```python
from build123d import *

# Parameters (mm, degrees)
F_3_0MM_DOWEL_HOLE1_D           = 3
F_3_0MM_DOWEL_HOLE1_ON_FACE_2_D = 3
SKETCH5_W                       = 1
SKETCH5_H                       = 1
AXIAL_TRANSMISION_DEPTH         = 2


with BuildPart() as part:
    # Sketch1 → Revolve1 (revolve)
    with BuildSketch(Plane(origin=(0, 0, 0), x_dir=(0, 0, -1), z_dir=(1, 0, 0))):
        with BuildLine():
            Line((15, 0), (15, 14))
            ThreePointArc((15, 14), (13.444368027, 22.077747211), (9, 29))
            ThreePointArc((9, 29), (6, 30.285714286), (3, 29))
            Line((3, 29), (3, 24))
            ThreePointArc((3, 24), (8.753905297, 20.403124237), (11, 14))
            Line((11, 14), (11, 0))
            Line((11, 0), (15, 0))
        make_face()
    revolve(axis=Axis((0, 0, -15), (0, 0, 1)))

    # Ø3.0mm Dowel Hole1 (through all)
    with Locations(Plane(origin=(0, 0, -15), x_dir=(0, -1, 0), z_dir=(0, 0, -1))):
        with Locations((0, 0)):
            Hole(F_3_0MM_DOWEL_HOLE1_D / 2)

    # Ø3.0mm Dowel Hole1 on face 2 (through all)
    with Locations(Plane(origin=(0, 0, 0), x_dir=(0, -1, 0), z_dir=(0, 0, -1))):
        with Locations((0, 0)):
            Hole(F_3_0MM_DOWEL_HOLE1_ON_FACE_2_D / 2)

    # Sketch5 → Axial_Transmision (cut)
    with BuildSketch(Plane.XY.offset(-11)):
        with Locations((0, 2.5)):
            Rectangle(SKETCH5_W, SKETCH5_H)
        with Locations((0, -2.5)):
            Rectangle(SKETCH5_W, SKETCH5_H)
    extrude(amount=-AXIAL_TRANSMISION_DEPTH, mode=Mode.SUBTRACT)


solid = part.part
```
Input: part model. Units: mm. Frame: model coordinates. Coordinates: 2 decimals unless noted, no trailing zeros. Write each loop counter-clockwise with the first axis right and the second up, starting at its lowest first coordinate (ties: lowest second). Pieces come first, ordered by that corner, then holes. Notation, with made-up numbers: (55, 44.5) -> (104, 44.5) arc R11 ccw to (104, 62.5) -> close; hole circle Ø8 at (-5, 31.25). An arc over 180 degrees is marked (long way). Answer as a JSON object with one key per item and string values.
1. Mould query, pull axis Y, two halves, no side actions, for faces 1 (the face through (3, 0, -11)), 2 (the face through (3, 0, -15)). Classes: released by +Y, released by -Y, zero draft, split by the parting line, or undercut.
Result set:
{"face 1": "undercut", "face 2": "zero draft"}
2. Material intervals for line 1 (Z direction, x = 10.5, y = -6); line 2 (X direction, y = 0, z = -13.1); line 3 (X direction, y = 0, z = -12.6), sorted ascending. Write a range as from..to.
Result set:
{"line 1": "z = -15..-11", "line 2": "x = -22.89..-1.5, 1.5..22.89", "line 3": "x = -23.93..-1.5, 1.5..23.93"}
3. Section A-A on z = -4.5. Return the cut outline in (x, y).
Result set:
{"outline": "circle Ø60.01 at (0, 0); hole circle Ø47.08 at (0, 0)"}
4. First-contact query: P1, Ø2, axis at x = 14.5, y = 10.5, coming from the +Z side; P2, Ø1.1, axis at x = 0, y = 2.5, coming from the +Z side; P3, Ø2, axis at x = 8, y = 20, coming from the -Z side. Flat tips, straight axial feed; report the tip coordinate or a pass-through.
Result set:
{"P1": "stops at z = -9.75", "P2": "stops at z = -11", "P3": "stops at z = -13.99"}
